Study the drawing (mm; zero at the part's minimum x, y, z) and answer. A direction names the side the tool comes from. Give positions to 0.01 mm unless a question says otherwise; leave off trailing zeros. Loops run counter-clockwise (first coordinate to the right, second up) from the corner with the lowest first, then second, coordinate; pieces in that order, holes last. Notation, with made-up numbers: M -11,57 L 29,57 A13 ccw 29,82 Z; hole C 0,-13.5 d3. An arc over 180 degrees is marked long. Return JSON: item names as keys, results as strings.
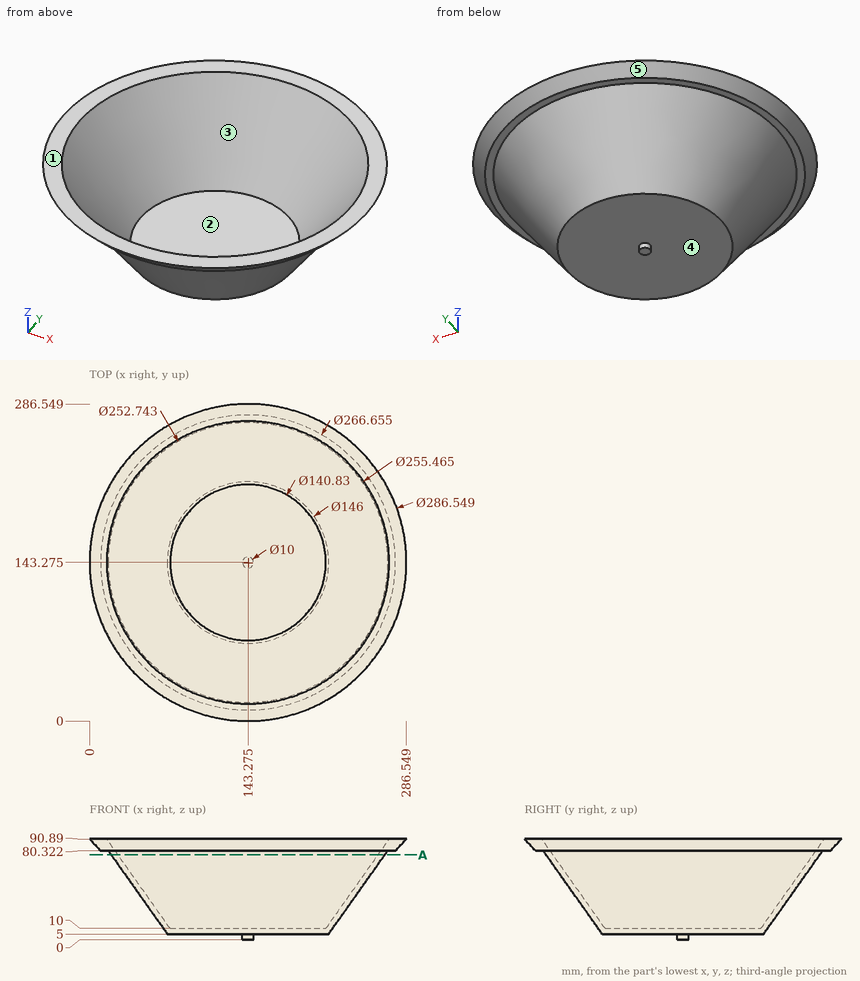
(1) Straight lines are drawn through the part: line 1 along Z through (x, y) = (97, 126); line 2 along X through (y, z) = (243, 72) (1 decimal); line 3 along X through (y, z) = (85.5, 68.5). For each, find the intervals that lie inside material, in ascending order.
Values follow:
{"line 1": "5 to 10", "line 2": "75.7 to 87.3, 199.2 to 210.9", "line 3": "40.39 to 47.48, 239.07 to 246.16"}
(2) A tool of negligible diameter and unlimited length cuts with its end or side. For the marked faces 1 and 2, from which of +Z, -Z, +X, -X, +Y, -Y can it reach the whole face along a straight path? Write none if from no direction.
Values follow:
{"face 1": "+Z, +X, -X, +Y, -Y", "face 2": "+Z"}
(3) The part is cut by section A-A (z = 76.5). Determine the outline of the cut face in (x, y) (1 decimal).
Values follow:
{"outline": "C 143.3,143.3 d247.3; hole C 143.3,143.3 d235.1"}
(4) Given pin 1 (1.5 mm diameter, centred on y = 194, z = 57, fed in from +X); pin 2 (4 mm diameter, centred on x = 160, y = 108, fed in from +Z); pin 3 (6 mm diameter, centred on x = 87.5, y = 88.5, fed in from -Z) (1 decimal), each flat-ended and moving along its own axis, determine where each tip first touches the part or whether it passes through.
Values follow:
{"pin 1": "x = 241.42", "pin 2": "z = 10", "pin 3": "z = 8.1"}
(5) Determine the mould class of the marked faces 3, 4 and 5 for opening direction X: released by +X, released by -X, zero draft, split by the parting line, or undercut.
Values follow:
{"face 3": "undercut", "face 4": "zero draft", "face 5": "split by the parting line"}
